```python
from build123d import *

# Parameters (mm, degrees)
SKETCH_1_W          = 19.5
SKETCH_1_H          = 8
EXTRUDE_1_DEPTH     = 5
FILLET_1_R          = 2.5
FILLET_2_R          = 0.5
CUT_EXTRUDE_2_DEPTH = 14.566963551
SKETCH_3_W          = 8.2
SKETCH_3_H          = 8
EXTRUDE_2_DEPTH     = 3
FILLET_3_R          = 3.5
SKETCH_4_R          = 3
CUT_EXTRUDE_3_DEPTH = 14.231118622


with BuildPart() as part:
    # 草图1 → 凸台-拉伸1 (new body)
    with BuildSketch(Plane.XY):
        Rectangle(SKETCH_1_W, SKETCH_1_H)
    extrude(amount=EXTRUDE_1_DEPTH)

    # 圆角1
    fillet_1_edges = [part.edges().sort_by_distance(p)[0] for p in [
        (-9.75, -4, 2.5),
        (9.75, 4, 2.5),
    ]]
    fillet(fillet_1_edges, radius=FILLET_1_R)

    # 圆角2
    fillet_2_edges = [part.edges().sort_by_distance(p)[0] for p in [
        (9.75, -4, 2.5),
        (-9.75, 4, 2.5),
    ]]
    fillet(fillet_2_edges, radius=FILLET_2_R)

    # 草图2 → 切除-拉伸2 (cut, through all)
    with BuildSketch(Plane.XZ.offset(4)):
        Polygon((-9.75, 2.5), (-6.914115374, 0), (-9.75, 0), align=None)
    cut_extrude_2 = extrude(amount=-CUT_EXTRUDE_2_DEPTH, mode=Mode.SUBTRACT)

    # 镜向1: 切除-拉伸2 across plane
    add(cut_extrude_2.mirror(Plane(origin=(0, 0, 0), x_dir=(0, 0, 1), z_dir=(1, 0, 0))), mode=Mode.SUBTRACT)

    # 草图3 → 凸台-拉伸2 (add)
    with BuildSketch(Plane.XY.offset(5)):
        Rectangle(SKETCH_3_W, SKETCH_3_H)
    extrude(amount=EXTRUDE_2_DEPTH)

    # 圆角3
    fillet_3_edges = [part.edges().sort_by_distance(p)[0] for p in [
        (4.1, -4, 6.5),
        (-4.1, 4, 6.5),
    ]]
    fillet(fillet_3_edges, radius=FILLET_3_R)

    # 草图4 → 切除-拉伸3 (cut, through all)
    with BuildSketch(Plane.XY.offset(8)):
        Circle(SKETCH_4_R)
    extrude(amount=-CUT_EXTRUDE_3_DEPTH, mode=Mode.SUBTRACT)


solid = part.part
```
For this review, take the finished solid that the model builds, in its own axes (mm). A direction names the side the tool comes from. Round coordinates to 2 decimals unless told otherwise and drop trailing zeros. Write each loop counter-clockwise with the first axis right and the second up, starting at its lowest first coordinate (ties: lowest second). Pieces come first, ordered by that corner, then holes.
1) Insertion check: pin 1 Ø1.5 at (y, z) = (-3, 6) entering from -X; pin 2 Ø1.5 at (y, z) = (2.5, 6.5) entering from +X; pin 3 Ø1 at (x, y) = (4.5, -2) entering from -Z. Each pin has a flat end and moves straight along its axis. Give the tip position at first contact, or say it passes through.
Answer below:
pin 1: stops at x = -4.1
pin 2: stops at x = 4.1
pin 3: stops at z = 0
2) Mouldability with a two-part tool opening along X and no side actions: class faces 5 (the face through (-3, 0, 4)), 6 (the face through (9.75, -1, 4)), 7 (the face through (1, -4, 3)), 8 (the face through (-9.75, 1, 4)) as +X half, -X half, draft (parallel to the pull), parting line (faces both ways), or undercut.
Answer below:
face 5: undercut
face 6: +X half
face 7: draft
face 8: -X half
3) For line 1 along Y through (x, z) = (0, 3); line 2 along Z through (x, y) = (4.75, -2.5); line 3 along X through (y, z) = (-2.5, 1.75), list the stretches that pass through material, from the lowest coordinate up.
Answer below:
line 1: y = -4 to -3, 3 to 4
line 2: z = 0 to 5
line 3: x = -8.9 to -1.66, 1.66 to 8.9
4) Take a section at A-A on x = 0. Give the boundary of the cut face in (y, z).
Answer below:
outline: (-4, 0) - (-3, 0) - (-3, 8) - (-4, 8) - close; (3, 0) - (4, 0) - (4, 8) - (3, 8) - close
5) Take a section at C-C on y = 0. Give the boundary of the cut face in (x, z).
Answer below:
outline: (-9.75, 2.5) - (-6.91, 0) - (-3, 0) - (-3, 8) - (-4.1, 8) - (-4.1, 5) - (-9.75, 5) - close; (3, 0) - (6.91, 0) - (9.75, 2.5) - (9.75, 5) - (4.1, 5) - (4.1, 8) - (3, 8) - close
6) Take a section at B-B on z = 4.75. Give the boundary of the cut face in (x, y), then the cut area to 3 significant figures.
Answer below:
outline: (-9.75, -1.5) arc R2.5 ccw to (-7.25, -4) - (9.25, -4) arc R0.5 ccw to (9.75, -3.5) - (9.75, 1.5) arc R2.5 ccw to (7.25, 4) - (-9.25, 4) arc R0.5 ccw to (-9.75, 3.5) - close; hole circle Ø6 at (0, 0)
area: 125 mm2
7) Take a section at D-D on z = 6.5. Give the boundary of the cut face in (x, y), then the cut area to 3 significant figures.
Answer below:
outline: (-4.1, -4) - (0.6, -4) arc R3.5 ccw to (4.1, -0.5) - (4.1, 4) - (-0.6, 4) arc R3.5 ccw to (-4.1, 0.5) - close; hole circle Ø6 at (0, 0)
area: 32.1 mm2
8) Machinability: for faces 1 (the face through (-4.1, -2, 6)), 2 (the face through (3.05, -3, 6.52)), 3 (the face through (4.1, 2, 6)), 4 (the face through (-3.05, 3, 6.52)), which of the approach directions +Z, -Z, +X, -X, +Y, -Y give a long, thin tool a straight path to every point of the face, cutting with its end or side? Answer none if there is none.
Answer below:
face 1: +Z, -X, +Y, -Y
face 2: +Z, +X, -Y
face 3: +Z, +X, +Y, -Y
face 4: +Z, -X, +Y
